```python
from build123d import *

# Parameters (mm, degrees)
BOX001_W        = 3
BOX001_H        = 4
BOX001_DEPTH    = 5
CHAMFER_SIZE    = 2
BOX002_W        = 2
BOX002_H        = 8
BOX002_DEPTH    = 3.725
CHAMFER001_SIZE = 1.8
SKETCH004_W     = 1
SKETCH004_H     = 14
PAD004_DEPTH    = 3.6
SKETCH005_W     = 28
SKETCH005_H     = 1
PAD005_DEPTH    = 3.6
SKETCH006_W     = 1
SKETCH006_H     = 14
PAD006_DEPTH    = 3.6
SKETCH003_W     = 28
SKETCH003_H     = 1
PAD003_DEPTH    = 3.6
BOX_W           = 28
BOX_H           = 14
BOX_DEPTH       = 0.125


with BuildPart() as chamfer_body:
    # Box001 → Box001 (new body)
    with BuildSketch(Plane(origin=(-1, 5, 0.125), x_dir=(1, 0, 0), z_dir=(0, 0, 1))):
        with Locations((1.5, 2)):
            Rectangle(BOX001_W, BOX001_H)
    extrude(amount=BOX001_DEPTH)

    # Chamfer
    chamfer_edges = [chamfer_body.edges().sort_by_distance(p)[0] for p in [
        (-1, 7, 0.125),
    ]]
    chamfer(chamfer_edges, length=CHAMFER_SIZE)


with BuildPart() as chamfer001:
    # Box002 → Box002 (new body)
    with BuildSketch(Plane(origin=(-2, 3, 0), x_dir=(1, 0, 0), z_dir=(0, 0, 1))):
        with Locations((1, 4)):
            Rectangle(BOX002_W, BOX002_H)
    extrude(amount=BOX002_DEPTH)

    # Chamfer001
    chamfer001_edges = [chamfer001.edges().sort_by_distance(p)[0] for p in [
        (-2, 3, 1.8625),
        (-2, 11, 1.8625),
    ]]
    chamfer(chamfer001_edges, length=CHAMFER001_SIZE)


with BuildPart() as pad004:
    # Sketch004 → Pad004 (new body)
    with BuildSketch(Plane.XY.offset(0.125)):
        with Locations((0.5, 7)):
            Rectangle(SKETCH004_W, SKETCH004_H)
    extrude(amount=PAD004_DEPTH)


with BuildPart() as pad005:
    # Sketch005 → Pad005 (new body)
    with BuildSketch(Plane.XY.offset(0.125)):
        with Locations((14, 0.5)):
            Rectangle(SKETCH005_W, SKETCH005_H)
    extrude(amount=PAD005_DEPTH)


with BuildPart() as pad006:
    # Sketch006 → Pad006 (new body)
    with BuildSketch(Plane.XY.offset(0.125)):
        with Locations((27.5, 7)):
            Rectangle(SKETCH006_W, SKETCH006_H)
    extrude(amount=PAD006_DEPTH)


with BuildPart() as walls:
    # Sketch003 → Pad003 (new body)
    with BuildSketch(Plane.XY.offset(0.125)):
        with Locations((14, 13.5)):
            Rectangle(SKETCH003_W, SKETCH003_H)
    extrude(amount=PAD003_DEPTH)

    # Fusion001: union Pad004, Pad005, Pad006
    add(pad004.part)
    add(pad005.part)
    add(pad006.part)

    # Fusion: union Chamfer001
    add(chamfer001.part)

    # Cut: cut Chamfer body
    add(chamfer_body.part, mode=Mode.SUBTRACT)


with BuildPart() as base_and_walls_do_not_edit:
    # Box → Box (new body)
    with BuildSketch(Plane.XY):
        with Locations((14, 7)):
            Rectangle(BOX_W, BOX_H)
    extrude(amount=BOX_DEPTH)

    # Fusion024: union Walls
    add(walls.part)


solid = base_and_walls_do_not_edit.part
```
CAD build for the part. Positions are in the model's coordinates, mm. A direction names the side the tool comes from. Round coordinates to 2 decimals unless told otherwise and drop trailing zeros. Order: outer loops, then holes, each group sorted by start corner. A loop starts at its lowest first (then second) coordinate and runs counter-clockwise, first axis right, second up.
Q1. Slice it at C-C (x = 25.5). Write the cut outline in (y, z) (3 decimals).
Q2. Wall check: L1, parallel to X at y = 6, z = 2.5; L2, parallel to Y at x = 7.75, z = 1.4; L3, parallel to X at y = 2.5, z = 3.4. Give the ranges that are in metal, low to high.
Q3. Slice it at A-A (z = 2.95). Write the cut outline in (x, y), and give its area (3 significant figures).
Q4. Drop flat-ended pins along their axis: pin 1 (2 mm diameter, centred on x = -0.5, z = 2, fed in from +Y); pin 2 (1.5 mm diameter, centred on y = 12, z = 2, fed in from -X); pin 3 (6 mm diameter, centred on x = 10, y = 6.5, fed in from +Z) (3 decimals). Give the stop position or say it passes through.
Q5. Two-plate mould, pull along Y, no slides. Class faces 4 (the flat face through (14, 14, 2)), 5 (the flat face through (14, 13, 2)), 6 (the flat face through (28, 7, 2)): pulls with the +Y half, pulls with the -Y half, needs draft (parallel to the pull), parting line crosses it, or undercut.
Q6. Slice it at B-B (y = 8.25). Write the cut outline in (x, z) (3 decimals), and give its area (4 significant figures).
Q7. Slice it at D-D (y = 3.5). Write the cut outline in (x, z) (3 decimals).
Q8. Which spindle directions (+Z, -Z, +X, -X, +Y, -Y) get a long thin tool onto all of the face, cutting with end or side? Do faces 1 (the flat face through (0, 12, 2)), 2 (the flat face through (27, 7, 2)), 3 (the flat face through (0, 1, 2)). Say none if no direction does.
Results below:
1. outline: (0, 0) - (14, 0) - (14, 3.725) - (13, 3.725) - (13, 0.125) - (1, 0.125) - (1, 3.725) - (0, 3.725) - close
2. L1: x = -2 to -1, 27 to 28
2. L2: y = 0 to 1, 13 to 14
2. L3: x = 0 to 1, 27 to 28
3. outline: (-2, 4.8) - (-0.2, 3) - (0, 3) - (0, 0) - (28, 0) - (28, 14) - (0, 14) - (0, 11) - (-0.2, 11) - (-2, 9.2) - close; hole (-1, 5) - (1, 5) - (1, 1) - (27, 1) - (27, 13) - (1, 13) - (1, 9) - (-1, 9) - close
3. area: 84.8 mm2
4. pin 1: stops at y = 14
4. pin 2: stops at x = 0
4. pin 3: stops at z = 0.125
5. face 4: pulls with the +Y half
5. face 5: undercut
5. face 6: needs draft
6. outline: (-2, 0) - (28, 0) - (28, 3.725) - (27, 3.725) - (27, 0.125) - (1, 0.125) - (-1, 2.125) - (-1, 3.725) - (-2, 3.725) - close
6. area: 12.95 mm2
7. outline: (-0.7, 0) - (28, 0) - (28, 3.725) - (27, 3.725) - (27, 0.125) - (1, 0.125) - (1, 3.725) - (-0.7, 3.725) - close
8. face 1: +Z, -Z, -X, +Y
8. face 2: +Z
8. face 3: +Z, -Z, -X, -Y
